Geometry check sheet. Reference: the model listing, model coordinates, mm. Face numbers are marked on the shaded views. Round coordinates to 2 decimals unless told otherwise and drop trailing zeros. Loops run counter-clockwise (first coordinate to the right, second up) from the corner with the lowest first, then second, coordinate; pieces in that order, holes last. Notation, with made-up numbers: M 36.25,14 L 90.25,14 A19 cw 90.25,30 Z; hole C -39.5,77.25 d3. An arc over 180 degrees is marked long. Write item = value, one per line.
Autodesk Fusion 360 part; units mm, degrees
sketch "Sketch1" plane through (0, 0, 0) normal (0, 1, 0) x (1, 0, 0)
  line L0 (0, 0) -> (30, 0)
  line L1 (30, 0) -> (30, 60)
  line L2 (30, 60) -> (40, 60)
  line L3 (40, 60) -> (40, 160)
  line L4 (40, 160) -> (0, 160)
  line L5 (0, 160) -> (0, 0)
  dimension "d8" = 100
  dimension "d9" = 160
  dimension "d10" = 30
revolve "Revolve1" add sketch "Sketch1" angle 360 about axis through (0, 0, -160) along (0, 0, 1)
fillet "Fillet1" radius 10 1 edges at (-37.2931, -14.4646, -60)
fillet "Fillet2" radius 15 1 edges at (-37.2931, -14.4646, -160)
shell "Shell1" thickness 2 removed faces 1 at (14.141, -6.0737, 0)
equation "overalheight = 160 mm"
equation "neckheight = 100 mm"
equation "fillet1 = 15 mm"
equation "fillet2 = 10 mm"
equation "fillet3 = 5 mm"
equation "diameter = 30 mm"
equation "wallthickness = 2 mm"
equation "d8 = neckheight"
equation "d9 = overalheight"
equation "d10 = diameter"
equation "d12 = fillet2"
equation "d13 = fillet1"
equation "d14 = wallthickness"
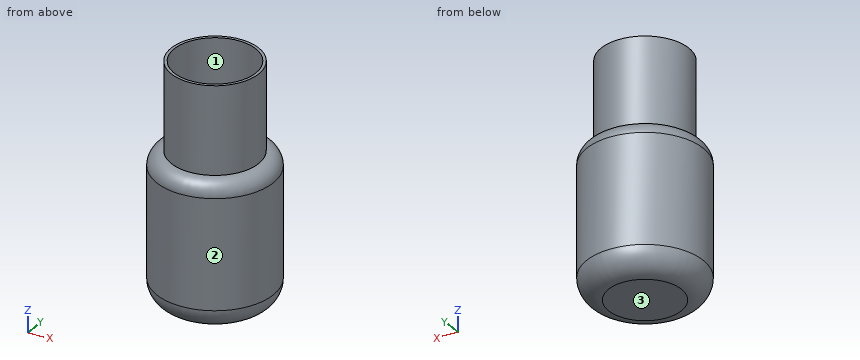
(1) Depth check by flat-ended pin: pin 1 Ø2 at (x, y) = (17, 29) entering from -Z; pin 2 Ø12 at (x, z) = (22.5, -56) entering from +Y; pin 3 Ø1 at (x, y) = (-6, 32) entering from -Z. Enter the tip coordinate at first touch or a pass-through.
Result set:
pin_1 = -157.92
pin_2 = 29
pin_3 = -158.24
(2) Sectioned sample at C-C on z = -18.5. Record the cut outline in (x, y).
Result set:
outline = C 0,0 d60; hole C 0,0 d56
(3) Material ranges on line 1 along Y through (x, z) = (0, -102.5); line 2 along Z through (x, y) = (-15.5, 4); line 3 along X through (y, z) = (33, -124), recorded low to high. Write a range as from..to.
Result set:
line_1 = -40..-38, 38..40
line_2 = -160..-158
line_3 = -22.61..-18.84, 18.84..22.61
(4) Release check for a two-part mould opening along Y. For the marked faces 1, 2 and 3 record: released by +Y, released by -Y, zero draft, split by the parting line, or undercut.
Result set:
face_1 = undercut
face_2 = split by the parting line
face_3 = zero draft
(5) Sectioned sample at D-D on z = -91.5. Record the cut outline in (x, y), then the cut area to 3 significant figures.
Result set:
outline = C 0,0 d80; hole C 0,0 d76
area = 490 mm2
